from build123d import *

# Parameters (mm, degrees)
CROQUIS1_W                    = 10
CROQUIS1_H                    = 18
SALIENTE_EXTRUIR1_DEPTH       = 6.35
TALADRO_ROSCADO_M4X0_71_D     = 3.3
DI_METRO_DE_TALADRO_5_0_5_1_D = 8


with BuildPart() as part:
    # Croquis1 → Saliente-Extruir1 (new, symmetric)
    with BuildSketch(Plane(origin=(0, 0, 0), x_dir=(0, 0, -1), z_dir=(1, 0, 0))):
        Rectangle(CROQUIS1_W, CROQUIS1_H)
    extrude(amount=SALIENTE_EXTRUIR1_DEPTH, both=True)

    # Taladro roscado M4x0.71 (through all)
    with Locations(Plane(origin=(6.35, 0, 0), x_dir=(0, 0, -1), z_dir=(1, 0, 0))):
        with Locations((0, 6), (0, -6)):
            Hole(TALADRO_ROSCADO_M4X0_71_D / 2)

    # Diámetro de taladro Ø5.0 (5)1 (through all)
    with Locations(Plane.XY.offset(5)):
        with Locations((0, 0)):
            Hole(DI_METRO_DE_TALADRO_5_0_5_1_D / 2)


solid = part.part
For this review, take the finished solid that the model builds, in its own axes (mm). Coordinates: 2 decimals unless noted, no trailing zeros. Order: outer loops, then holes, each group sorted by start corner. A loop starts at its lowest first (then second) coordinate and runs counter-clockwise, first axis right, second up. Notation, with made-up numbers: (54, 4.5) - (77, 4.5) arc R7 ccw to (77, 9.5) - close; hole circle Ø6 at (18, -34.5). An arc over 180 degrees is marked (long way). Answer as CSV lines item,"result". Start each with the question number.
1) Draft analysis for pull direction Z (two halves, no side actions). For faces 1 (the cylindrical face through (0.867, -3.905, -0.07)), 2 (the cylindrical face through (-0.1, -7.6, -0.4)), 3 (the flat face through (-1.3, -4.1, 5)), state which applies: +Z half, -Z half, draft (parallel to the pull), parting line (faces both ways), or undercut.
2) Insertion check: P1, Ø3, axis at y = 6, z = 0, coming from the -X side. The pin has a flat end and moves straight along its axis. Give the tip position at first contact, or say it passes through.
3) To check wall thickness, follow line 1 along Y through (x, z) = (0, 0); line 2 along Y through (x, z) = (-5.25, 0); line 3 along Y through (x, z) = (4.5, -1.25). State the ranges of each line that lie inside material, in increasing order. Write a range as [from, to].
4) Add section C-C (z = 0). State the section outline as (x, y) points.
5) Add section A-A (x = 0). State the section outline as (y, z) points, then the cut area to 3 significant figures.
6) Add section B-B (y = 0). State the section outline as (x, z) points, then the cut area to 3 significant figures.
7) Add section D-D (x = 5). State the section outline as (y, z) points.
Result:
1,face 1,"draft"
1,face 2,"undercut"
1,face 3,"+Z half"
2,P1,"through"
3,line 1,"[-9, -7.65], [-4.35, -4], [4, 4.35], [7.65, 9]"
3,line 2,"[-9, -7.65], [-4.35, 4.35], [7.65, 9]"
3,line 3,"[-9, -7.08], [-4.92, 4.92], [7.08, 9]"
4,outline,"(-6.35, -9) - (6.35, -9) - (6.35, -7.65) - (-6.35, -7.65) - close; (-6.35, -4.35) - (6.35, -4.35) - (6.35, 4.35) - (-6.35, 4.35) - close; (-6.35, 7.65) - (6.35, 7.65) - (6.35, 9) - (-6.35, 9) - close; hole circle Ø8 at (0, 0)"
5,outline,"(-9, -5) - (-4, -5) - (-4, 5) - (-9, 5) - close; (4, -5) - (9, -5) - (9, 5) - (4, 5) - close; hole circle Ø3.3 at (-6, 0); hole circle Ø3.3 at (6, 0)"
5,area,"82.9 mm^2"
6,outline,"(-6.35, -5) - (-4, -5) - (-4, 5) - (-6.35, 5) - close; (4, -5) - (6.35, -5) - (6.35, 5) - (4, 5) - close"
6,area,"47.0 mm^2"
7,outline,"(-9, -5) - (9, -5) - (9, 5) - (-9, 5) - close; hole circle Ø3.3 at (-6, 0); hole circle Ø3.3 at (6, 0)"
